Part model, mm, in its own coordinate system. Give positions to 0.01 mm unless a question says otherwise; leave off trailing zeros. Order: outer loops, then holes, each group sorted by start corner. A loop starts at its lowest first (then second) coordinate and runs counter-clockwise, first axis right, second up. Notation, with made-up numbers: (39.25, 46) -> (57.25, 46) arc R26 ccw to (57.25, 76) -> close; hole circle Ø7 at (12.5, -17). An arc over 180 degrees is marked (long way). Write item = value, one per line. Start each with the question number.
Item 1: Band-saw the part on C-C on y = -3. Count the separate pieces of the cut face and the enclosed holes in it, plus the area to 3 significant figures.
Item 2: Flat gauge pins, fed straight in: P1, Ø4, axis at x = -337.5, y = -2, coming from the +Z side; P2, Ø1, axis at y = -1, z = 88.5, coming from the -X side. Where does each tip first touch, or does it go through?
Item 3: Pull direction Z, two halves, no side cores. Call faces 1 (the face through (-152.86, -4.06, 83.73)), 2 (the face through (-5, -8, -2)): +Z half, -Z half, draft (parallel to the pull), parting line (faces both ways), or undercut.
Item 4: Band-saw the part on B-B on x = 66.5. Write the cut outline in (y, z), plus the area to 3 significant figures.
Item 5: Band-saw the part on A-A on z = -89. Write the cut outline in (x, y), plus the area to 3 significant figures.
Item 6: Drill centre lines: line 1 along Z through (x, y) = (66.5, -3.25); line 2 along X through (y, z) = (-5.75, 89); line 3 along X through (y, z) = (-3.75, 0.5). Where is each one in solid material? Low to high.
```python
from build123d import *

# Parameters (mm, degrees)
SKETCH1_W                        = 685
SKETCH1_H                        = 250
BASE_FLANGE1_DEPTH               = 8
SKETCH6_W                        = 60
SKETCH6_H                        = 8
SKETCH6_W_2                      = 70
EXTRUDE1_DEPTH                   = 8
SKETCH7_W                        = 250
SKETCH7_H                        = 73.5
BASE_FLANGE2_DEPTH               = 8
SKETCH12_W                       = 30.5
SKETCH12_H                       = 8.5
EXTRUDE2_DEPTH                   = 699.681794525
SKETCH14_W                       = 250
SKETCH14_H                       = 8
BASE_FLANGE3_DEPTH               = 50.5
SKETCH19_W                       = 60
SKETCH19_H                       = 8
SKETCH19_W_2                     = 70
EXTRUDE3_DEPTH                   = 8
BREAK_CORNER1_START              = 41.5
BREAK_CORNER1_DEPTH              = 8
EXTRUDE4_DEPTH                   = 8
BASE_FLANGE4_DEPTH               = 8
SKETCH38_W                       = 8.5
SKETCH38_H                       = 20.5
EXTRUDE5_DEPTH                   = 10
SKETCH39_W                       = 20.5
SKETCH39_H                       = 8.5
EXTRUDE6_DEPTH                   = 10
F_12_5_12_5_DIAMETER_HOLE1_D     = 12.5
F_12_5_12_5_DIAMETER_HOLE1_DEPTH = 10
F_12_5_12_5_DIAMETER_HOLE1_TIP   = 3.755378869


# Read off the part's stored shape, not the designer's step: Break-Corner1
# Sheet-metal steps are written as plain solids
with BuildPart() as part:
    # Sketch1 → Base-Flange1 (new body)
    with BuildSketch(Plane(origin=(0, 0, 0), x_dir=(1, 0, 0), z_dir=(0, 1, 0))):
        Rectangle(SKETCH1_W, SKETCH1_H)
    extrude(amount=-BASE_FLANGE1_DEPTH)

    # Sketch6 → Extrude1 (cut)
    with BuildSketch(Plane(origin=(342.5, 0, 0), x_dir=(0, 0, -1), z_dir=(1, 0, 0))):
        with Locations((-95, -4)):
            Rectangle(SKETCH6_W, SKETCH6_H)
        with Locations((95, -4)):
            Rectangle(SKETCH6_W, SKETCH6_H)
        with Locations((0, -4)):
            Rectangle(SKETCH6_W_2, SKETCH6_H)
    extrude1 = extrude(amount=-EXTRUDE1_DEPTH, mode=Mode.SUBTRACT)

    # Mirror1: Extrude1 across plane
    add(extrude1.mirror(Plane(origin=(0, 0, 0), x_dir=(0, 0, 1), z_dir=(1, 0, 0))), mode=Mode.SUBTRACT)

    # Sketch39 → Extrude6 (cut)
    with BuildSketch(Plane.XZ.offset(8)):
        with Locations((289.5, 0)):
            Rectangle(SKETCH39_W, SKETCH39_H)
        with Locations((229.5, 0)):
            Rectangle(SKETCH39_W, SKETCH39_H)
        with Locations((-289.5, 0)):
            Rectangle(SKETCH39_W, SKETCH39_H)
        with Locations((-229.5, 0)):
            Rectangle(SKETCH39_W, SKETCH39_H)
    extrude(amount=-EXTRUDE6_DEPTH, mode=Mode.SUBTRACT)

    # Ø12.5 (12.5) Diameter Hole1
    with Locations(Plane(origin=(131.975, 0, 2029.150100001), x_dir=(1, 0, 0), z_dir=(0, 1, 0))):
        with Locations((-281.475, 2118.150100001), (-281.475, 1940.150100001), (-65.475, 1940.150100001), (-65.475, 2118.150100001)):
            Hole(F_12_5_12_5_DIAMETER_HOLE1_D / 2, depth=F_12_5_12_5_DIAMETER_HOLE1_DEPTH)
            with Locations((0, 0, -(F_12_5_12_5_DIAMETER_HOLE1_DEPTH + F_12_5_12_5_DIAMETER_HOLE1_TIP / 2))):  # 118° drill point
                Cone(0, F_12_5_12_5_DIAMETER_HOLE1_D / 2, F_12_5_12_5_DIAMETER_HOLE1_TIP, mode=Mode.SUBTRACT)


with BuildPart() as body_2:
    # Sketch7 → Base-Flange2 (new body)
    with BuildSketch(Plane(origin=(334.5, 0, 0), x_dir=(0, 0, -1), z_dir=(1, 0, 0))):
        with Locations((0, 20.75)):
            Rectangle(SKETCH7_W, SKETCH7_H)
    extrude(amount=BASE_FLANGE2_DEPTH)

    # Sketch12 → Extrude2 (cut, through all)
    with BuildSketch(Plane(origin=(342.5, 0, 0), x_dir=(0, 0, -1), z_dir=(1, 0, 0))):
        with Locations((-50, -4)):
            Rectangle(SKETCH12_W, SKETCH12_H)
        with Locations((50, -4)):
            Rectangle(SKETCH12_W, SKETCH12_H)
        with Locations((50, 45.5)):
            Rectangle(SKETCH12_W, SKETCH12_H)
        with Locations((-50, 45.5)):
            Rectangle(SKETCH12_W, SKETCH12_H)
    extrude(amount=-EXTRUDE2_DEPTH, mode=Mode.SUBTRACT)

    # Sketch38 → Extrude5 (cut)
    with BuildSketch(Plane(origin=(342.5, 0, 0), x_dir=(0, 0, -1), z_dir=(1, 0, 0))):
        with Locations((0, 27.5)):
            Rectangle(SKETCH38_W, SKETCH38_H)
    extrude(amount=-EXTRUDE5_DEPTH, mode=Mode.SUBTRACT)


with BuildPart() as body_3:
    # Sketch14 → Base-Flange3 (new body)
    with BuildSketch(Plane.ZY.offset(-334.5)):
        with Locations((0, 45.5)):
            Rectangle(SKETCH14_W, SKETCH14_H)
    extrude(amount=-BASE_FLANGE3_DEPTH)

    # Sketch19 → Extrude3 (cut)
    with BuildSketch(Plane(origin=(342.5, 0, 0), x_dir=(0, 0, -1), z_dir=(1, 0, 0))):
        with Locations((95, 45.5)):
            Rectangle(SKETCH19_W, SKETCH19_H)
        with Locations((0, 45.5)):
            Rectangle(SKETCH19_W_2, SKETCH19_H)
        with Locations((-95, 45.5)):
            Rectangle(SKETCH19_W, SKETCH19_H)
    extrude(amount=-EXTRUDE3_DEPTH, mode=Mode.SUBTRACT)

    # Break-Corner1 outline → Break-Corner1 (cut)
    with BuildSketch(Plane(origin=(0, 0, 0), x_dir=(1, 0, 0), z_dir=(0, 1, 0)).offset(BREAK_CORNER1_START)):
        Polygon((385, -125), (385, -110), (370, -125), align=None)
        Polygon((370, 125), (385, 110), (385, 125), align=None)
    extrude(amount=BREAK_CORNER1_DEPTH, mode=Mode.SUBTRACT)

    # Sketch20 → Extrude4 (cut)
    with BuildSketch(Plane(origin=(0, 49.5, 0), x_dir=(1, 0, 0), z_dir=(0, 1, 0))):
        with BuildLine():
            Line((367, 75), (367, 55))
            ThreePointArc((367, 55), (362.5, 50.5), (358, 55))
            Line((358, 55), (358, 75))
            ThreePointArc((358, 75), (362.5, 79.5), (367, 75))
        make_face()
        with BuildLine():
            Line((367, -75), (367, -55))
            ThreePointArc((367, -55), (362.5, -50.5), (358, -55))
            Line((358, -55), (358, -75))
            ThreePointArc((358, -75), (362.5, -79.5), (367, -75))
        make_face()
    extrude(amount=-EXTRUDE4_DEPTH, mode=Mode.SUBTRACT)


with BuildPart() as body_4:
    # Mirror4: mirrored copy
    add(body_3.part.mirror(Plane(origin=(0, 0, 0), x_dir=(0, 0, 1), z_dir=(1, 0, 0))))


with BuildPart() as body_5:
    # Sketch29 → Base-Flange4 (new body)
    with BuildSketch(Plane.XY.offset(4)):
        Polygon((219.5, 0), (219.5, -8), (239.5, -8), (239.5, 0), (279.5, 0), (279.5, -8), (299.5, -8), (299.5, 0), (334.5, 0), (334.5, 17.5), (342.5, 17.5), (342.5, 37.5), (334.5, 37.5), (334.5, 57.5), (194.5, 10), (194.5, 0), align=None)
    extrude(amount=-BASE_FLANGE4_DEPTH)


with BuildPart() as body_6:
    # Mirror5: mirrored copy
    add(body_5.part.mirror(Plane(origin=(0, 0, 0), x_dir=(0, 0, 1), z_dir=(1, 0, 0))))


with BuildPart() as body_7:
    # Mirror3: mirrored copy
    add(body_2.part.mirror(Plane(origin=(0, 0, 0), x_dir=(0, 0, 1), z_dir=(1, 0, 0))))


solid = part.part
```
Values found:
q1.separate_pieces = 1
q1.enclosed_holes = 8
q1.area = 167,000 mm^2
q2.P1 = 65
q2.P2 = -334.5
q3.face_1 = undercut
q3.face_2 = draft
q4.outline = (-8, -125) -> (0, -125) -> (0, -95.25) -> (-8, -95.25) -> close; (-8, -82.75) -> (0, -82.75) -> (0, 82.75) -> (-8, 82.75) -> close; (-8, 95.25) -> (0, 95.25) -> (0, 125) -> (-8, 125) -> close
q4.area = 1,800 mm^2
q5.outline = (-334.5, -8) -> (-155.75, -8) -> (-155.75, 0) -> (-334.5, 0) -> close; (-143.25, -8) -> (60.25, -8) -> (60.25, 0) -> (-143.25, 0) -> close; (72.75, -8) -> (334.5, -8) -> (334.5, 0) -> (72.75, 0) -> close
q5.area = 5,150 mm^2
q6.line_1 = -125 to -95.25, -82.75 to 82.75, 95.25 to 125
q6.line_2 = -334.5 to -155.75, -143.25 to 60.25, 72.75 to 334.5
q6.line_3 = -334.5 to -299.75, -279.25 to -239.75, -219.25 to 219.25, 239.75 to 279.25, 299.75 to 334.5
